Geometry: final body of the model. Coordinates: model frame, mm. Face numbers are marked on the shaded views. A direction names the side the tool comes from. Give positions to 0.01 mm unless a question says otherwise; leave off trailing zeros. Order: outer loops, then holes, each group sorted by start corner. A loop starts at its lowest first (then second) coordinate and runs counter-clockwise, first axis right, second up. Notation, with made-up numbers: (35, 13) - (91, 13) arc R11 cw to (91, 23) - close; hole circle Ø9 at (9, -38.5). An arc over 180 degrees is marked (long way). Put each result on its own line as item: value. Start each with the question number.
1. Set-up query: the marked faces 1, 2 and 3. Return all of +Z, -Z, +X, -X, +Y, -Y with unobstructed straight access to the full face (end or side cutting, diameter ignored); none if empty.
2. Section C-C on x = 14.5. Return the cut outline in (y, z), plus the area to 3 significant figures.
3. Ray query, line 1 along X through (y, z) = (1, -27); line 2 along Z through (x, y) = (12.75, 2.65). Return the intervals inside material, ascending. Write a range as from..to.
4. Section A-A on z = -2. Return the cut outline in (x, y), plus the area to 3 significant figures.
5. Section B-B on y = 4.4. Return the cut outline in (x, z).
6. Mould query, pull axis X, two halves, no side actions, for the marked faces 4, 5 and 6. Classes: pulls with the +X half, pulls with the -X half, needs draft (parallel to the pull), parting line crosses it, or undercut.
7. First-contact query: P1, Ø2.5, axis at y = 4, z = -2, coming from the -X side; P2, Ø2.5, axis at x = 15.5, y = 1.5, coming from the -Z side. Flat tips, straight axial feed; report the tip coordinate or a pass-through.
from build123d import *

# Parameters (mm, degrees)
SKETCH1_W           = 30
SKETCH1_H           = 30.88
BOSS_EXTRUDE1_DEPTH = 5.44
CAVITY1_START       = 10
CAVITY1_OUTLINE_W   = 5.44
CAVITY1_OUTLINE_H   = 5.44
CAVITY1_DEPTH       = 10


# Read off the part's stored shape, not the designer's step: Cavity1
with BuildPart() as part:
    # Sketch1 → Boss-Extrude1 (new body)
    with BuildSketch(Plane(origin=(0, 0, 0), x_dir=(1, 0, 0), z_dir=(0, 1, 0))):
        with Locations((15, 15.44)):
            Rectangle(SKETCH1_W, SKETCH1_H)
    extrude(amount=BOSS_EXTRUDE1_DEPTH)

    # Cavity1 outline → Cavity1 (cut)
    with BuildSketch(Plane.YZ.offset(CAVITY1_START)):
        with Locations((2.72, -28.16)):
            Rectangle(CAVITY1_OUTLINE_W, CAVITY1_OUTLINE_H)
        with Locations((2.72, -2.72)):
            Rectangle(CAVITY1_OUTLINE_W, CAVITY1_OUTLINE_H)
    extrude(amount=CAVITY1_DEPTH, mode=Mode.SUBTRACT)


solid = part.part
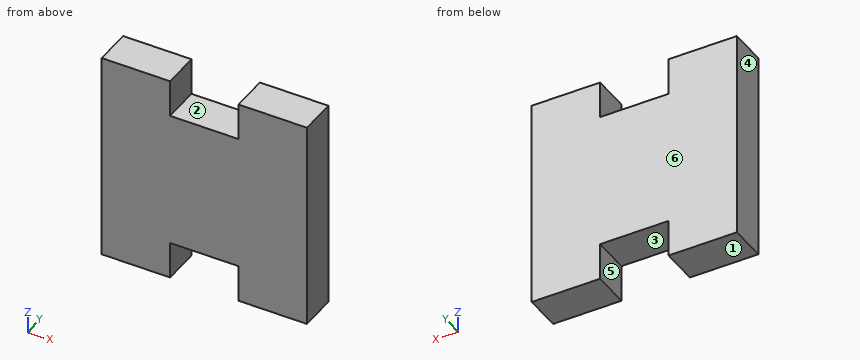
Resolved:
1. face 1: -Z, +X, -X, +Y, -Y
1. face 2: +Z, +Y, -Y
1. face 3: -Z, +Y, -Y
2. outline: (0, -25.44) - (5.44, -25.44) - (5.44, -5.44) - (0, -5.44) - close
2. area: 109 mm^2
3. line 1: 0..10, 20..30
3. line 2: -25.44..-5.44
4. outline: (0, 0) - (10, 0) - (10, 5.44) - (0, 5.44) - close; (20, 0) - (30, 0) - (30, 5.44) - (20, 5.44) - close
4. area: 109 mm^2
5. outline: (0, -30.88) - (10, -30.88) - (10, -25.44) - (20, -25.44) - (20, -30.88) - (30, -30.88) - (30, 0) - (20, 0) - (20, -5.44) - (10, -5.44) - (10, 0) - (0, 0) - close
6. face 4: pulls with the -X half
6. face 5: undercut
6. face 6: needs draft
7. P1: x = 0
7. P2: z = -25.44
